from build123d import *

# Parameters (mm, degrees)
SKETCH_1_W      = 42.7
SKETCH_1_H      = 21
SKETCH_1_R      = 1.5
EXTRUDE_1_DEPTH = 2
SKETCH_2_R      = 1.25
SKETCH_2_R_2    = 3
EXTRUDE_2_DEPTH = 2


with BuildPart() as part:
    # 草图1 → 凸台-拉伸1 (new body)
    with BuildSketch(Plane(origin=(0, 0, 0), x_dir=(1, 0, 0), z_dir=(0, 1, 0))):
        Rectangle(SKETCH_1_W, SKETCH_1_H)
        with Locations(Location((7.5, 5, 0), (0, 0, 270))):
            Circle(SKETCH_1_R, mode=Mode.SUBTRACT)
        with Locations(Location((7.5, -5, 0), (0, 0, 90))):
            Circle(SKETCH_1_R, mode=Mode.SUBTRACT)
        with Locations(Location((-7.5, -5, 0), (0, 0, 270))):
            Circle(SKETCH_1_R, mode=Mode.SUBTRACT)
        with Locations(Location((-7.5, 5, 0), (0, 0, 90))):
            Circle(SKETCH_1_R, mode=Mode.SUBTRACT)
        with BuildLine():
            Line((8.017950723, 1.550908082), (12.912587519, 1.550908082))
            ThreePointArc((12.912587519, 1.550908082), (14.126270768, 1.145131224), (14.697546856, 0))
            ThreePointArc((14.697546856, 0), (14.126270768, -1.145131224), (12.912587519, -1.550908082))
            Line((12.912587519, -1.550908082), (8.017950723, -1.550908082))
            add(Edge.make_bspline(
                [(0, -7.407271614), (2.092471107, -7.358009404), (3.043739342, -2.951912586), (6.007732496, -1.626733157), (8.017950723, -1.550908082)],
                knots=[0, 0, 0, 0, 0.496822763, 1, 1, 1, 1], degree=3))
            add(Edge.make_bspline(
                [(0, -7.407271614), (-2.092471107, -7.358009404), (-3.043739342, -2.951912586), (-6.007732496, -1.626733157), (-8.017950723, -1.550908082)],
                knots=[0, 0, 0, 0, 0.496822763, 1, 1, 1, 1], degree=3))
            Line((-8.017950723, -1.550908082), (-12.912587519, -1.550908082))
            ThreePointArc((-12.912587519, -1.550908082), (-14.126270768, -1.145131224), (-14.697546856, 0))
            ThreePointArc((-14.697546856, 0), (-14.126270768, 1.145131224), (-12.912587519, 1.550908082))
            Line((-12.912587519, 1.550908082), (-8.017950723, 1.550908082))
            add(Edge.make_bspline(
                [(0, 7.407271614), (-2.092471107, 7.358009404), (-3.043739342, 2.951912586), (-6.007732496, 1.626733157), (-8.017950723, 1.550908082)],
                knots=[0, 0, 0, 0, 0.496822763, 1, 1, 1, 1], degree=3))
            add(Edge.make_bspline(
                [(0, 7.407271614), (2.092471107, 7.358009404), (3.043739342, 2.951912586), (6.007732496, 1.626733157), (8.017950723, 1.550908082)],
                knots=[0, 0, 0, 0, 0.496822763, 1, 1, 1, 1], degree=3))
        make_face(mode=Mode.SUBTRACT)
    extrude(amount=EXTRUDE_1_DEPTH)

    # 草图2 → 凸台-拉伸2 (add)
    with BuildSketch(Plane.ZY.offset(21.35)):
        with BuildLine():
            Line((-10.5, 2), (-10.5, 46))
            ThreePointArc((-10.5, 46), (0, 56.5), (10.5, 46))
            Line((10.5, 46), (10.5, 2))
            Line((10.5, 2), (-10.5, 2))
        make_face()
        with Locations((0, 38.65)):
            Circle(SKETCH_2_R, mode=Mode.SUBTRACT)
        with Locations((-7.35, 46)):
            Circle(SKETCH_2_R, mode=Mode.SUBTRACT)
        with Locations((0, 53.35)):
            Circle(SKETCH_2_R, mode=Mode.SUBTRACT)
        with Locations((7.35, 46)):
            Circle(SKETCH_2_R, mode=Mode.SUBTRACT)
        with Locations((0, 46)):
            Circle(SKETCH_2_R_2, mode=Mode.SUBTRACT)
        with BuildLine():
            Line((-2.091438456, 33.71946821), (-2.091438456, 8.682620376))
            ThreePointArc((-2.091438456, 8.682620376), (-4.622608783, 10.734209017), (-5.574745456, 13.850179963))
            Line((-5.574745456, 13.850179963), (-5.574745456, 28.551908623))
            ThreePointArc((-5.574745456, 28.551908623), (-4.622608783, 31.667879569), (-2.091438456, 33.71946821))
        make_face(mode=Mode.SUBTRACT)
        with BuildLine():
            Line((5.574745456, 28.551908623), (5.574745456, 13.850179963))
            ThreePointArc((5.574745456, 13.850179963), (4.622608783, 10.734209017), (2.091438456, 8.682620376))
            Line((2.091438456, 8.682620376), (2.091438456, 33.71946821))
            ThreePointArc((2.091438456, 33.71946821), (4.622608783, 31.667879569), (5.574745456, 28.551908623))
        make_face(mode=Mode.SUBTRACT)
    extrude_2 = extrude(amount=-EXTRUDE_2_DEPTH)

    # 镜向1: 凸台-拉伸2 across plane
    add(extrude_2.mirror(Plane(origin=(0, 0, 0), x_dir=(0, 0, 1), z_dir=(1, 0, 0))))


solid = part.part
The listing builds one solid part. Answer for the finished solid, in the listing's coordinates (mm). A direction names the side the tool comes from. Give positions to 0.01 mm unless a question says otherwise; leave off trailing zeros. Write each loop counter-clockwise with the first axis right and the second up, starting at its lowest first coordinate (ties: lowest second). Pieces come first, ordered by that corner, then holes. Notation, with made-up numbers: (17, 58.5) -> (44, 58.5) arc R18 cw to (44, 73.5) -> close; hole circle Ø6 at (0, -1). An arc over 180 degrees is marked (long way). Use a Markdown table: item, result.
(1) Section A-A, the plane y = 7.5 is taken. Determine the outline of the cut face in (x, z), then the cut area to 3 significant figures.
Return value:
| item | result |
|---|---|
| outline | (-21.35, -10.5) -> (-19.35, -10.5) -> (-19.35, 10.5) -> (-21.35, 10.5) -> close; (19.35, -10.5) -> (21.35, -10.5) -> (21.35, 10.5) -> (19.35, 10.5) -> close |
| area | 84.0 mm2 |
(2) For faces 1 (the flat face through (10, 1, -1.551)), 2 (the flat face through (20, 21, 5.575)), 3 (the flat face through (0, 1, 10.5)), determine the directions among +Z, -Z, +X, -X, +Y, -Y from which every point of the face is accessible in a straight line to the end or side of a thin tool.
Return value:
| item | result |
|---|---|
| face 1 | +Y, -Y |
| face 2 | +X, -X |
| face 3 | +Z, +X, -X, +Y, -Y |
(3) Section D-D, the plane y = 18.5 is taken. Determine the outline of the cut face in (x, z).
Return value:
| item | result |
|---|---|
| outline | (-21.35, -10.5) -> (-19.35, -10.5) -> (-19.35, -5.57) -> (-21.35, -5.57) -> close; (-21.35, -2.09) -> (-19.35, -2.09) -> (-19.35, 2.09) -> (-21.35, 2.09) -> close; (-21.35, 5.57) -> (-19.35, 5.57) -> (-19.35, 10.5) -> (-21.35, 10.5) -> close; (19.35, -10.5) -> (21.35, -10.5) -> (21.35, -5.57) -> (19.35, -5.57) -> close; (19.35, -2.09) -> (21.35, -2.09) -> (21.35, 2.09) -> (19.35, 2.09) -> close; (19.35, 5.57) -> (21.35, 5.57) -> (21.35, 10.5) -> (19.35, 10.5) -> close |
(4) Flat-ended cylindrical pins translate along their axes: P1, Ø1.5, axis at y = 46, z = 7.35, coming from the -X side; P2, Ø6, axis at x = -14, z = -7.5, coming from the +Y side; P3, Ø5, axis at x = -7.5, z = 8, coming from the -Y side. Find the tip coordinate at first contact, or state that the pin passes through.
Return value:
| item | result |
|---|---|
| P1 | through |
| P2 | y = 2 |
| P3 | y = 0 |
(5) Section C-C, the plane y = 38.65 is taken. Determine the outline of the cut face in (x, z).
Return value:
| item | result |
|---|---|
| outline | (-21.35, -10.5) -> (-19.35, -10.5) -> (-19.35, -1.25) -> (-21.35, -1.25) -> close; (-21.35, 1.25) -> (-19.35, 1.25) -> (-19.35, 10.5) -> (-21.35, 10.5) -> close; (19.35, -10.5) -> (21.35, -10.5) -> (21.35, -1.25) -> (19.35, -1.25) -> close; (19.35, 1.25) -> (21.35, 1.25) -> (21.35, 10.5) -> (19.35, 10.5) -> close |
(6) Section B-B, the plane x = -11.5 is taken. Determine the outline of the cut face in (y, z).
Return value:
| item | result |
|---|---|
| outline | (0, -10.5) -> (2, -10.5) -> (2, -1.55) -> (0, -1.55) -> close; (0, 1.55) -> (2, 1.55) -> (2, 10.5) -> (0, 10.5) -> close |
(7) Determine the mould class of faces 4 (the cylindrical face through (-20.4, 56.5, -0.2)), 5 (the flat face through (19.35, 30, 0)), 6 (the cylindrical face through (-14.14, 0.986, -1.133)) for opening direction X: released by +X, released by -X, zero draft, split by the parting line, or undercut.
Return value:
| item | result |
|---|---|
| face 4 | zero draft |
| face 5 | undercut |
| face 6 | undercut |
(8) Find the intervals of material crossed by probe 1 along Y at (x, z) = (-20.6, 0); probe 2 along X at (y, z) = (44.5, 5.25); probe 3 along Y at (x, z) = (-14.5, -1.25), in increasing order. Write a range as from..to.
Return value:
| item | result |
|---|---|
| probe 1 | 0..37.4, 39.9..43, 49..52.1, 54.6..56.5 |
| probe 2 | -21.35..-19.35, 19.35..21.35 |
| probe 3 | 0..2 |
